Here's the drawing with two shaded views (mm, measured from the low corner). I have some questions. Give positions to 0.01 mm unless a question says otherwise; leave off trailing zeros. Write each loop counter-clockwise with the first axis right and the second up, starting at its lowest first coordinate (ties: lowest second). Pieces come first, ordered by that corner, then holes. Notation, with made-up numbers: (-25, 82.5) -> (-12, 82.5) arc R21 ccw to (-12, 112.5) -> close; hole circle Ø11 at (23, -32). An arc over 180 degrees is marked (long way). One line per question, with ' | ' between items.
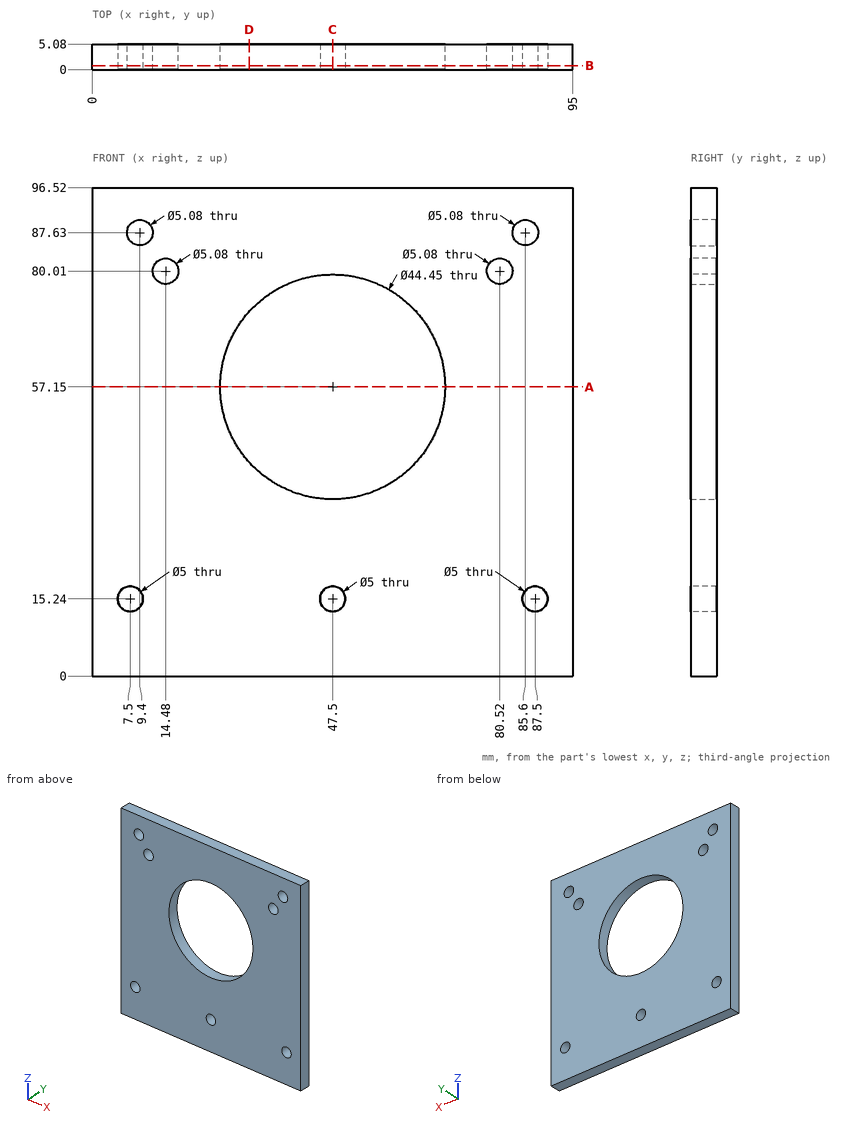
Q1. If I drill on line 1 along X through (y, z) = (2.8, 87.63); line 2 along X through (y, z) = (0.3, 89); line 3 along Z through (x, y) = (7.5, 3.6), over which ranges is the centre line in solid material (lowest first)?
Answer below:
line 1: x = 0 to 6.86, 11.94 to 83.06, 88.14 to 95 | line 2: x = 0 to 7.26, 11.54 to 83.46, 87.74 to 95 | line 3: z = 0 to 12.74, 17.74 to 85.94, 89.32 to 96.52
Q2. Will these pins go through, and if not, where does the flat tip stop? pin 1 (3 mm diameter, centred on x = 7.5, z = 15.24, fed in from +Y); pin 2 (2 mm diameter, centred on x = 82.5, z = 52, fed in from -Y).
Answer below:
pin 1: passes through | pin 2: stops at y = 0
Q3. Imagine slicing it at C-C on x = 47.5. Please give me the cut outline in (y, z) (3 decimals), and give its area (3 significant figures).
Answer below:
outline: (0, 0) -> (5.08, 0) -> (5.08, 12.74) -> (0, 12.74) -> close; (0, 17.74) -> (5.08, 17.74) -> (5.08, 34.925) -> (0, 34.925) -> close; (0, 79.375) -> (5.08, 79.375) -> (5.08, 96.52) -> (0, 96.52) -> close | area: 239 mm^2
Q4. Imagine slicing it at D-D on x = 31. Please give me the cut outline in (y, z), and give its area (3 significant figures).
Answer below:
outline: (0, 0) -> (5.08, 0) -> (5.08, 42.26) -> (0, 42.26) -> close; (0, 72.04) -> (5.08, 72.04) -> (5.08, 96.52) -> (0, 96.52) -> close | area: 339 mm^2
Q5. Imagine slicing it at A-A on z = 57.15. Please give me the cut outline in (x, y) (3 decimals), and give its area (3 significant figures).
Answer below:
outline: (0, 0) -> (25.275, 0) -> (25.275, 5.08) -> (0, 5.08) -> close; (69.725, 0) -> (95, 0) -> (95, 5.08) -> (69.725, 5.08) -> close | area: 257 mm^2
Q6. Imagine slicing it at B-B on y = 0.8. Count the separate pieces of the cut face and the enclosed holes in it, and give its area (3 significant figures).
Answer below:
separate pieces: 1 | enclosed holes: 8 | area: 7,480 mm^2
